Geometry check sheet. Reference: the model listing, model coordinates, mm. A direction names the side the tool comes from. Round coordinates to 2 decimals unless told otherwise and drop trailing zeros. Write each loop counter-clockwise with the first axis right and the second up, starting at its lowest first coordinate (ties: lowest second). Pieces come first, ordered by that corner, then holes. Notation, with made-up numbers: M -22.75,32 L -11.75,32 A22 cw -11.75,62 Z; hole C 42.5,-13 d10. An arc over 180 degrees is marked long. Put each result on its own line as item: value. Start each with the question number.
(1) Section check C-C on z = -33. Record the cut outline in (x, y), then the cut area to 3 significant figures.
(2) Mould release check, pull along X, two halves, no side actions. Record for faces 1 (the flat face through (-97.389, -75.487, -31.868)), 2 (the flat face through (-111, -56, -28.826)), 3 (the flat face through (-61.12, -111.92, -31.87)): pulls with the +X half, pulls with the -X half, needs draft (parallel to the pull), parting line crosses it, or undercut.
(3) Gauge pin test, flat ends, axial feed: pin 1 (1.5 mm diameter, centred on y = -30.5, z = -30.5, fed in from +X); pin 2 (2 mm diameter, centred on x = -107, z = -29.5, fed in from +Y); pin 3 (4.5 mm diameter, centred on x = 27.34, y = -44.83, fed in from +Z). Record the tip position at first contact, or that the pin passes through.
(4) Section check A-A on y = -2. Record the cut outline in (x, z).
(5) Tool access check on faces 4 (the flat face through (-41.78, 38.16, -31.87)), 5 (the flat face through (-5.51, 1.72, -31.87)). Record the directions out of +Z, -Z, +X, -X, +Y, -Y that give a thin tool (end or side, any length) a straight path to the whole face; none if there is none.
(6) Material ranges on probe 1 along X at (y, z) = (-43, -29.55); probe 2 along Y at (x, z) = (25, -34.3); probe 3 along Y at (x, z) = (-59.5, -32.85), recorded low to high.
(7) Section check B-B on x = 11. Record the cut outline in (y, z).
Autodesk Inventor part; units mm, degrees
ref_plane "YZ Plane" through (0, 0, 0) normal (1, 0, 0) x (0, 1, 0)
ref_plane "XZ Plane" through (0, 0, 0) normal (0, 1, 0) x (-1, 0, 0)
ref_plane "XY Plane" through (0, 0, 0) normal (0, 0, 1) x (1, 0, 0)
ref_plane "Work Plane1" through (-43.297, -16.1171, -34.8261) normal (0, 0, 1) x (0.7745, 0.6326, 0)
sketch "Sketch1" plane through (-43.297, -16.1171, -34.8261) normal (0, 0, 1) x (0.7745, 0.6326, 0)
  line L0 (-79.4504, 49.077) -> (40.5496, 49.077)
  line L1 (40.5496, 49.077) -> (40.5496, -70.923)
  line L2 (40.5496, -70.923) -> (-79.4504, -70.923)
  line L3 (-79.4504, -70.923) -> (-79.4504, 49.077)
  line L4 (-77.4504, 47.077) -> (38.5496, 47.077)
  line L5 (38.5496, 47.077) -> (38.5496, -68.923)
  line L6 (38.5496, -68.923) -> (-77.4504, -68.923)
  line L7 (-77.4504, -68.923) -> (-77.4504, 47.077)
  line L8 (-79.4504, 49.077) -> (-71.4504, 49.077)
  line L9 (-71.4504, 49.077) -> (-71.4504, 41.077)
  line L10 (-71.4504, 41.077) -> (-79.4504, 41.077)
  line L11 (-79.4504, 41.077) -> (-79.4504, 49.077)
  line L12 (40.5496, 49.077) -> (32.5496, 49.077)
  line L13 (32.5496, 49.077) -> (32.5496, 41.077)
  line L14 (32.5496, 41.077) -> (40.5496, 41.077)
  line L15 (40.5496, 41.077) -> (40.5496, 49.077)
  line L16 (-79.4504, -70.923) -> (-71.4504, -70.923)
  line L17 (-71.4504, -70.923) -> (-71.4504, -62.923)
  line L18 (-71.4504, -62.923) -> (-79.4504, -62.923)
  line L19 (-79.4504, -62.923) -> (-79.4504, -70.923)
  line L20 (40.5496, -70.923) -> (32.5496, -70.923)
  line L21 (32.5496, -70.923) -> (32.5496, -62.923)
  line L22 (32.5496, -62.923) -> (40.5496, -62.923)
  line L23 (40.5496, -62.923) -> (40.5496, -70.923)
  circle A0 centre (-75.4504, 45.077) radius 2
  circle A1 centre (36.5496, 45.077) radius 2
  circle A2 centre (-75.4504, -66.923) radius 2
  circle A3 centre (36.5496, -66.923) radius 2
  point P0 (43.7284, -14.9068)
  point P1 (-71.4504, 47.077)
  point P2 (32.5496, 47.077)
  point P3 (38.5496, 41.077)
  point P4 (38.5496, -62.923)
  point P5 (32.5496, -68.923)
  point P6 (-71.4504, -68.923)
  point P7 (-77.4504, -62.923)
  point P8 (-77.4504, 41.077)
  dimension "d0" = 2
  dimension "d1" = 120
  dimension "d2" = 120
  dimension "d3" = 8
  dimension "d4" = 8
  dimension "d5" = 8
  dimension "d6" = 8
  dimension "d7" = 8
  dimension "d8" = 8
  dimension "d9" = 8
  dimension "d10" = 8
  dimension "d11" = 4
  dimension "d12" = 4
  dimension "d13" = 4
  dimension "d14" = 4
  dimension "d15" = 4
  dimension "d16" = 4
  dimension "d17" = 4
  dimension "d18" = 4
  dimension "d19" = 4
  dimension "d20" = 4
  dimension "d21" = 4
  dimension "d22" = 4
extrude "Extrusion1" add sketch "Sketch1" along normal blind 6 contours L0 L9 L4 L7 L10 L3 | L0 L13 L4 L9 | L10 L7 L18 L3 | L0 L1 L14 L5 L4 L13 | L9 L10 L7 A0 L4 | L18 L7 L6 L17 L2 L3 | L4 A1 L5 L14 L13 | A0 L7 L4 | L18 L17 L6 A2 L7 | L1 L22 L5 L14 | L4 L5 A1 | L17 L6 L21 L2 | A2 L6 L7 | L1 L2 L21 L6 L5 L22 | L5 A3 L6 L21 L22 | L5 L6 A3
equation "\"d2\" = d1"
equation "\"d3\" = d6"
equation "\"d4\" = d6"
equation "\"d5\" = d6"
equation "\"d7\" = d6"
equation "\"d8\" = d6"
equation "\"d9\" = d6"
equation "\"d10\" = d6"
equation "\"d15\" = d18"
equation "\"d16\" = d17"
equation "\"d18\" = d17"
equation "\"d19\" = d17"
equation "\"d20\" = d17"
equation "\"d21\" = d17"
equation "\"d22\" = d17"
properties part number "Stage_shunt"
Answers follow:
1. outline: M -135.88,-28.37 L -59.97,-121.31 L 32.97,-45.39 L -42.94,47.54 Z; hole C -130.25,-28.93 d4; hole M -129.27,-33.3 L -63.48,-113.84 L -58.83,-110.05 L -55.03,-114.7 L 25.51,-48.91 L 21.72,-44.26 L 26.36,-40.46 L -39.43,40.08 L -44.07,36.29 L -47.87,40.93 L -128.41,-24.86 L -124.62,-29.5 Z; hole C -59.4,-115.68 d4; hole C -43.51,41.92 d4; hole C 27.34,-44.83 d4
1. area: 1,040 mm^2
2. face 1: pulls with the -X half
2. face 2: needs draft
2. face 3: undercut
3. pin 1: stops at x = 21.42
3. pin 2: stops at y = -3.96
3. pin 3: stops at z = -28.83
4. outline: M -103.59,-34.83 L -100.43,-34.83 L -100.43,-28.83 L -103.59,-28.83 Z; M -5.05,-34.83 L -2.47,-34.83 L -2.47,-28.83 L -5.05,-28.83 Z
5. face 4: +Z, -Z
5. face 5: +Z, -Z, +X, +Y
6. probe 1: x = -123.92 to -121.34, 23.26 to 26.53, 28.16 to 31.02
6. probe 2: y = -51.91 to -49.32, -48.28 to -41.58, -38.79 to -35.63
6. probe 3: y = -120.93 to -117.67, -113.68 to -110.6, 31.43 to 34.02
7. outline: M -63.34,-34.83 L -60.76,-34.83 L -60.76,-28.83 L -63.34,-28.83 Z; M -21.65,-34.83 L -18.49,-34.83 L -18.49,-28.83 L -21.65,-28.83 Z
